Source: CAD feature listing. Evaluate the final solid. Frame: model axes, mm. A direction names the side the tool comes from. Give positions to 0.01 mm unless a question says otherwise; leave off trailing zeros. Write each loop counter-clockwise with the first axis right and the second up, starting at its lowest first coordinate (ties: lowest second). Pieces come first, ordered by that corner, then holes.
```python
from build123d import *

# Parameters (mm, degrees)
SKETCH1_W                = 87
SKETCH1_H                = 66
SKETCH1_R                = 1.375
BOSS_EXTRUDE1_DEPTH      = 10
CUT_EXTRUDE1_DEPTH       = 56.509008278
CUT_EXTRUDE1_DEPTH_BACK  = 56.509008278
BOSS_EXTRUDE2_DEPTH      = 43.5
BOSS_EXTRUDE2_DEPTH_BACK = 43.5
SKETCH3_W                = 5
SKETCH3_H                = 20
CUT_EXTRUDE2_DEPTH       = 10


with BuildPart() as part:
    # Sketch1 → Boss-Extrude1 (new body)
    with BuildSketch(Plane(origin=(0, 0, 0), x_dir=(1, 0, 0), z_dir=(0, 1, 0))):
        Rectangle(SKETCH1_W, SKETCH1_H)
        with Locations(Location((-40, 24.5, 0), (0, 0, 270))):
            Circle(SKETCH1_R, mode=Mode.SUBTRACT)
        with Locations(Location((-40, -24.5, 0), (0, 0, 270))):
            Circle(SKETCH1_R, mode=Mode.SUBTRACT)
        with Locations(Location((18, 24.5, 0), (0, 0, 270))):
            Circle(SKETCH1_R, mode=Mode.SUBTRACT)
        with Locations(Location((18, -24.5, 0), (0, 0, 270))):
            Circle(SKETCH1_R, mode=Mode.SUBTRACT)
    extrude(amount=BOSS_EXTRUDE1_DEPTH)

    # Sketch2 → Cut-Extrude1 (cut, two sides: drawn at the far end of the back side and taken through both)
    with BuildSketch(Plane(origin=(0, 0, 0), x_dir=(0, 0, -1), z_dir=(1, 0, 0)).offset(-CUT_EXTRUDE1_DEPTH_BACK)):
        Polygon((33, 5), (3, 5), (8, 0), (33, 0), align=None)
        Polygon((-33, 5), (-3, 5), (-8, 0), (-33, 0), align=None)
    extrude(amount=CUT_EXTRUDE1_DEPTH + CUT_EXTRUDE1_DEPTH_BACK, mode=Mode.SUBTRACT)

    # Sketch3 → Boss-Extrude2 (add, two sides: drawn at the far end of the back side and taken through both)
    with BuildSketch(Plane(origin=(0, 0, 0), x_dir=(0, 0, -1), z_dir=(1, 0, 0)).offset(-BOSS_EXTRUDE2_DEPTH_BACK)):
        with Locations((30.5, 20)):
            Rectangle(SKETCH3_W, SKETCH3_H)
        with Locations((-30.5, 20)):
            Rectangle(SKETCH3_W, SKETCH3_H)
    extrude(amount=BOSS_EXTRUDE2_DEPTH + BOSS_EXTRUDE2_DEPTH_BACK)

    # Sketch4 → Cut-Extrude2 (cut)
    with BuildSketch(Plane.XY.offset(33)):
        Polygon((-26.5, 17), (-26.5, 20.250689265), (17.5, 20.250689265), (17.5, 10), (-26.5, 10), (-38.5, 10), (-38.5, 17), align=None)
    extrude(amount=-CUT_EXTRUDE2_DEPTH, mode=Mode.SUBTRACT)


solid = part.part
```
1. Cut plane B-B, the plane x = -40. Return the cut outline in (y, z) (3 decimals).
2. Cut plane D-D, the plane x = -8. Return the cut outline in (y, z).
3. Cut plane A-A, the plane y = 14.5. Return the cut outline in (x, z).
4. Line query: L1, parallel to X at y = 7.6, z = -24.5 (3 decimals); L2, parallel to Z at x = 18, y = 6.5 (3 decimals); L3, parallel to Z at x = -26.5, y = 25. Output: solid intervals per line, ascending.
5. Contact query for flat-ended pins moving along their axis: P1, Ø4, axis at x = 4, z = 31.5, coming from the -Y side; P2, Ø1.5, axis at x = -2, z = 4, coming from the +Y side; P3, Ø1, axis at x = 5.5, y = 18, coming from the +Z side. Output: stop coordinate, or through.
6. Mould query, pull axis X, two halves, no side actions, for faces 4 (the flat face through (-1, 5, -18)), 5 (the flat face through (-43.5, 9, 0)), 6 (the flat face through (-26.5, 19, 31)). Classes: +X half, -X half, draft (parallel to the pull), parting line (faces both ways), or undercut.
7. Access query for faces 1 (the flat face through (-33, 17, 31)), 2 (the flat face through (-1, 22, 28)), 3 (the cylindrical face through (18.929, 7.465, 23.487)). Directions: +Z, -Z, +X, -X, +Y, -Y. A direction counts if a zero-diameter tool reaches every point of the face in a straight line with its end or side. Return the directions, or none.
8. Cut plane C-C, the plane z = 24.5. Return the cut outline in (x, y) (3 decimals), then the cut area to 4 significant figures.
Response values:
1. outline: (0, -8) - (5, -3) - (5, -23.125) - (10, -23.125) - (10, 23.125) - (5, 23.125) - (5, 3) - (0, 8) - close; (5, -33) - (30, -33) - (30, -28) - (10, -28) - (10, -25.875) - (5, -25.875) - close; (5, 25.875) - (10, 25.875) - (10, 28) - (30, 28) - (30, 33) - (5, 33) - close
2. outline: (0, -8) - (5, -3) - (5, -33) - (30, -33) - (30, -28) - (10, -28) - (10, 33) - (5, 33) - (5, 3) - (0, 8) - close; (20.25, 28) - (30, 28) - (30, 33) - (20.25, 33) - close
3. outline: (-43.5, -33) - (43.5, -33) - (43.5, -28) - (-43.5, -28) - close; (-43.5, 28) - (-38.5, 28) - (-38.5, 33) - (-43.5, 33) - close; (17.5, 28) - (43.5, 28) - (43.5, 33) - (17.5, 33) - close
4. L1: x = -43.5 to -41.375, -38.625 to 16.625, 19.375 to 43.5
4. L2: z = -33 to -25.875, -23.125 to 23.125, 25.875 to 33
4. L3: z = -33 to -28, 28 to 33
5. P1: stops at y = 5
5. P2: stops at y = 10
5. P3: stops at z = -28
6. face 4: draft
6. face 5: -X half
6. face 6: undercut
7. face 1: +Z
7. face 2: +X, -X, +Y
7. face 3: +Y, -Y
8. outline: (-43.5, 5) - (-41.375, 5) - (-41.375, 10) - (-43.5, 10) - close; (-38.625, 5) - (16.625, 5) - (16.625, 10) - (-38.625, 10) - close; (19.375, 5) - (43.5, 5) - (43.5, 10) - (19.375, 10) - close
8. area: 407.5 mm2
